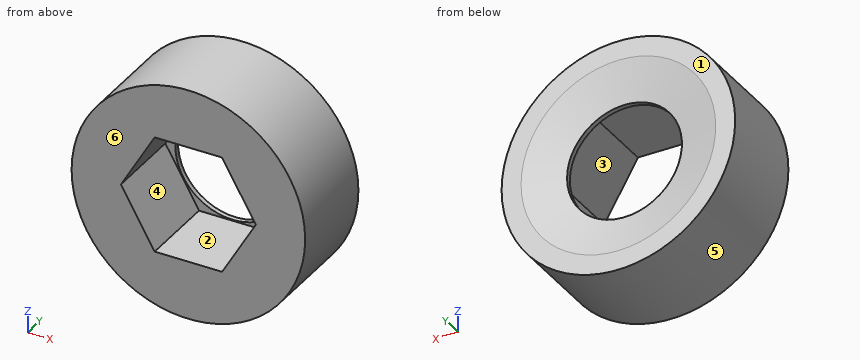
```python
from build123d import *

# Parameters (mm, degrees)
SKETCH1_R           = 12
BOSS_EXTRUDE1_DEPTH = 8
SKETCH2_R           = 12
SKETCH2_R_2         = 5.9
BOSS_EXTRUDE2_DEPTH = 1.6
SKETCH3_R           = 10
CUT_EXTRUDE1_DEPTH  = 1.1
CUT_EXTRUDE1_TAPER  = 75


with BuildPart() as part:
    # Sketch1 → Boss-Extrude1 (new body)
    with BuildSketch(Plane(origin=(0, 0, 0), x_dir=(1, 0, 0), z_dir=(0, 1, 0))):
        Circle(SKETCH1_R)
        Polygon((3.464101615, 6), (-3.464101615, 6), (-6.92820323, 0), (-3.464101615, -6), (3.464101615, -6), (6.92820323, 0), align=None, mode=Mode.SUBTRACT)
    extrude(amount=BOSS_EXTRUDE1_DEPTH)

    # Sketch2 → Boss-Extrude2 (add)
    with BuildSketch(Plane(origin=(0, 8, 0), x_dir=(1, 0, 0), z_dir=(0, 1, 0))):
        Circle(SKETCH2_R)
        Circle(SKETCH2_R_2, mode=Mode.SUBTRACT)
    extrude(amount=BOSS_EXTRUDE2_DEPTH)

    # Sketch3 → Cut-Extrude1 (cut)
    with BuildSketch(Plane(origin=(0, 9.6, 0), x_dir=(1, 0, 0), z_dir=(0, 1, 0))):
        Circle(SKETCH3_R)
    extrude(amount=-CUT_EXTRUDE1_DEPTH, taper=CUT_EXTRUDE1_TAPER, mode=Mode.SUBTRACT)


solid = part.part
```
Work out the finished part from the listing and answer in its coordinate system (mm). Face numbers are marked on the shaded views. A direction names the side the tool comes from. Coordinates: 2 decimals unless noted, no trailing zeros. Order: outer loops, then holes, each group sorted by start corner. A loop starts at its lowest first (then second) coordinate and runs counter-clockwise, first axis right, second up. Notation, with made-up numbers: (69.25, 88.5) - (102.25, 88.5) arc R31 cw to (102.25, 115.5) - close; hole circle Ø5 at (-20, 66.25). An arc over 180 degrees is marked (long way). Answer as a JSON object with one key per item and string values.
1. The mould has two halves that part along X. Classify the marked faces 3, 4, 5 and 6: +X half, -X half, draft (parallel to the pull), parting line (faces both ways), or undercut.
Output values:
{"face 3": "undercut", "face 4": "undercut", "face 5": "parting line", "face 6": "draft"}
2. Find section A-A on x = 0. Determine the outline of the cut face in (y, z), plus the area to 3 significant figures.
Output values:
{"outline": "(0, -12) - (9.6, -12) - (9.6, -10) - (8.5, -5.9) - (8, -5.9) - (8, -6) - (0, -6) - close; (0, 6) - (8, 6) - (8, 5.9) - (8.5, 5.9) - (9.6, 10) - (9.6, 12) - (0, 12) - close", "area": "111 mm²"}
3. Consider line 1 (Z direction, x = 0, y = 8.1); line 2 (Z direction, x = 0, y = 1). Determine where each line is inside the solid, lowest interval first.
Output values:
{"line 1": "z = -12 to -5.9, 5.9 to 12", "line 2": "z = -12 to -6, 6 to 12"}
4. Each of these flat-tipped pins is pushed along its axis until it touches: P1, Ø2, axis at y = 3, z = -4.5, coming from the -X side; P2, Ø10, axis at x = 5.5, z = -4, coming from the +Y side; P3, Ø2, axis at x = -9.5, y = 6, coming from the -Z side; P4, Ø3, axis at x = -8.5, y = 5, coming from the +Z side. Where does it stop, or does it pass through?
Output values:
{"P1": "stops at x = -11.48", "P2": "stops at y = 9.6", "P3": "stops at z = -8.47", "P4": "stops at z = 9.75"}
5. A tool of negligible diameter and unlimited length cuts with its end or side. For the marked faces 1 and 2, from which of +Z, -Z, +X, -X, +Y, -Y can it reach the whole face along a straight path? Write none if from no direction.
Output values:
{"face 1": "+Z, -Z, +X, -X, +Y", "face 2": "-Y"}
6. Find section B-B on y = 7.25. Determine the outline of the cut face in (x, z), plus the area to 3 significant figures.
Output values:
{"outline": "circle Ø24 at (0, 0); hole (-6.93, 0) - (-3.46, -6) - (3.46, -6) - (6.93, 0) - (3.46, 6) - (-3.46, 6) - close", "area": "328 mm²"}
